Design review of the part shown in the three views and the two pictorial views. Dimensions are in mm from the part's minimum x, y and z. A direction names the side the tool comes from. Coordinates: 2 decimals unless noted, no trailing zeros. Order: outer loops, then holes, each group sorted by start corner. A loop starts at its lowest first (then second) coordinate and runs counter-clockwise, first axis right, second up. Notation, with made-up numbers: (-28.5, 87) -> (0.5, 87) arc R5 ccw to (0.5, 94) -> close; hole circle Ø10 at (-17, 22.5). An arc over 180 degrees is marked (long way). Answer as a JSON object with one key per item and string values. Group by question number.
1) Add section C-C, the plane y = 23.25. Write out the cut boundary in (x, z), then the cut area to 3 significant figures.
2) Add section A-A, the plane x = 52.2. Write out the cut boundary in (y, z), then the cut area to 3 significant figures.
3) Add section D-D, the plane z = 17. Write out the cut boundary in (x, y).
4) Machinability: for the marked faces 4, 5, 6, 7 and 8, which of the approach directions +Z, -Z, +X, -X, +Y, -Y give a long, thin tool a straight path to every point of the face, cutting with its end or side? Answer none if there is none.
5) For pin 1 (5 mm diameter, centred on x = 58, y = 20, fed in from -Z); pin 2 (3 mm diameter, centred on x = 66.5, z = 16.5, fed in from +Y); pin 3 (1.8 mm diameter, centred on y = 7, z = 8, fed in from -X); pin 4 (5 mm diameter, centred on y = 11.5, z = 8.5, fed in from -X), all flat-tipped, find the tip position at first contact; note any pin that passes through.
6) Draft analysis for pull direction X (two halves, no side actions). For the marked faces 1, 2 and 3, state which applies: +X half, -X half, draft (parallel to the pull), parting line (faces both ways), or undercut.
7) Add section B-B, the plane z = 2.25. Write out the cut boundary in (x, y), then the cut area to 3 significant figures.
8) Wall thickness on L1, parallel to X at y = 22.25, z = 8.75; L2, parallel to X at y = 11.75, z = 11.75; L3, parallel to Y at x = 14.5, z = 10: over which ranges is each line inside the solid? List them lowest first.
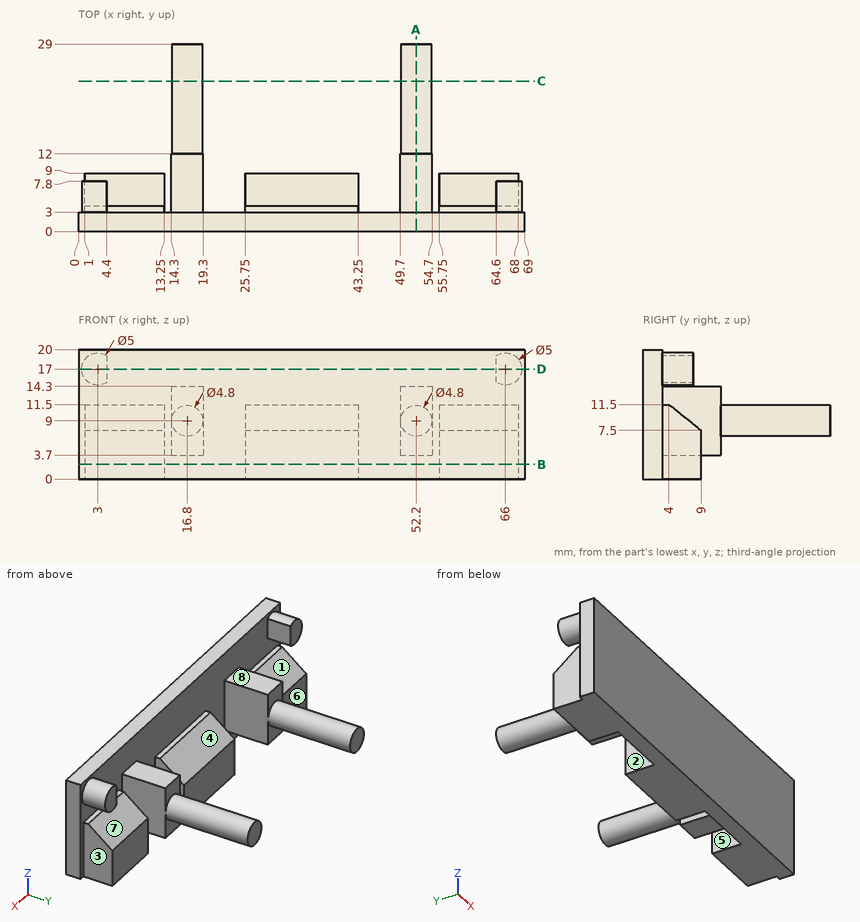
Output values:
{
 "1": {"outline": "circle Ø4.8 at (16.8, 9); circle Ø4.8 at (52.2, 9)", "area": "36.2 mm²"},
 "2": {"outline": "(0, 0) -> (3, 0) -> (3, 3.7) -> (12, 3.7) -> (12, 6.6) -> (29, 6.6) -> (29, 11.4) -> (12, 11.4) -> (12, 14.3) -> (3, 14.3) -> (3, 20) -> (0, 20) -> close", "area": "237 mm²"},
 "3": {"outline": "(0, 0) -> (69, 0) -> (69, 3) -> (68.5, 3) -> (68.5, 7.8) -> (64.6, 7.8) -> (64.6, 3) -> (4.4, 3) -> (4.4, 7.8) -> (0.5, 7.8) -> (0.5, 3) -> (0, 3) -> close"},
 "4": {"face 4": "+Z, +Y", "face 5": "+Z, -Z, +Y", "face 6": "+Z, -Z, -X, +Y", "face 7": "+X, +Y", "face 8": "+Z, +X, -X, +Y"},
 "5": {"pin 1": "passes through", "pin 2": "stops at y = 7.8", "pin 3": "stops at x = 1", "pin 4": "stops at x = 14.3"},
 "6": {"face 1": "draft", "face 2": "undercut", "face 3": "+X half"},
 "7": {"outline": "(0, 0) -> (69, 0) -> (69, 3) -> (68, 3) -> (68, 9) -> (55.75, 9) -> (55.75, 3) -> (43.25, 3) -> (43.25, 9) -> (25.75, 9) -> (25.75, 3) -> (13.25, 3) -> (13.25, 9) -> (1, 9) -> (1, 3) -> (0, 3) -> close", "area": "459 mm²"},
 "8": {"L1": "x = 14.41 to 19.19, 49.81 to 54.59", "L2": "x = 14.3 to 19.3, 49.7 to 54.7", "L3": "y = 0 to 12"}
}
